```python
from build123d import *

# Parameters (mm, degrees)
SKETCH_W    = 80
SKETCH_H    = 88
SKETCH_R    = 9.5
SKETCH_R_2  = 3
PAD_DEPTH   = 10
FILLET_R    = 1
FILLET001_R = 10


with BuildPart() as part:
    # Sketch → Pad (new body)
    with BuildSketch(Plane.XY):
        with Locations((15, -15)):
            Rectangle(SKETCH_W, SKETCH_H)
        with Locations((0, -30)):
            Circle(SKETCH_R, mode=Mode.SUBTRACT)
        with Locations((-10, -52)):
            Circle(SKETCH_R_2, mode=Mode.SUBTRACT)
        with Locations((40, -52)):
            Circle(SKETCH_R_2, mode=Mode.SUBTRACT)
        with Locations((40, 22)):
            Circle(SKETCH_R_2, mode=Mode.SUBTRACT)
        with Locations((-10, 22)):
            Circle(SKETCH_R_2, mode=Mode.SUBTRACT)
        with BuildLine():
            ThreePointArc((-5, -6.244998), (8, 0), (-5, 6.244998))
            Line((-5, 9), (-5, 6.244998))
            Line((-8.125, 9), (-5, 9))
            Line((-8.125, -9), (-8.125, 9))
            Line((-5, -9), (-8.125, -9))
            Line((-5, -6.244998), (-5, -9))
        make_face(mode=Mode.SUBTRACT)
    extrude(amount=PAD_DEPTH)

    # Fillet
    fillet_edges = [part.edges().sort_by_distance(p)[0] for p in [
        (55, -59, 5),
        (55, 29, 5),
    ]]
    fillet(fillet_edges, radius=FILLET_R)

    # Fillet001
    fillet001_edges = [part.edges().sort_by_distance(p)[0] for p in [
        (-25, -59, 5),
        (-25, 29, 5),
    ]]
    fillet(fillet001_edges, radius=FILLET001_R)


solid = part.part
```
The model under review builds one solid part; all positions refer to its coordinate system, in mm. A direction names the side the tool comes from. Coordinates: 2 decimals unless noted, no trailing zeros. Write each loop counter-clockwise with the first axis right and the second up, starting at its lowest first coordinate (ties: lowest second). Pieces come first, ordered by that corner, then holes. Notation, with made-up numbers: (53, 19) -> (62, 19) arc R19 ccw to (62, 44) -> close; hole circle Ø9 at (-20, 70.5). An arc over 180 degrees is marked (long way). One line per item, written item: value. Start each with the question number.
Q1. Add section A-A, the plane y = 0. Give the boundary of the cut face in (x, z) (3 decimals), then the cut area to 3 significant figures.
Q2. To check wall thickness, follow probe 1 along Y at (x, z) = (0, 7); probe 2 along Y at (x, z) = (-4, 4.5); probe 3 along X at (y, z) = (0, 3.25) (3 decimals). State the ranges of each line that lie inside material, in increasing order.
Q3. Add section B-B, the plane x = 40. Give the boundary of the cut face in (y, z), then the cut area to 3 significant figures.
Q4. Add section D-D, the plane y = 22. Give the boundary of the cut face in (x, z), then the cut area to 3 significant figures.
Q5. Add section C-C, the plane z = 5.75. Give the boundary of the cut face in (x, y) (3 decimals).
Q6. Clearance check with a flat-ended pin moving along its axis: P1, Ø9.5, axis at x = 40, y = 22, coming from the -Z side. State where the tip first meets the part, or that it passes through.
Q7. The part is to be moulded in two halves that separate along X. For faces 1 (the face through (55, -16, 5)), 2 (the face through (-22.15, 25.99, 5.07)), 3 (the face through (14, -14, 0)), 4 (the face through (37.79, -49.97, 4.93)), say which applies: +X half, -X half, draft (parallel to the pull), parting line (faces both ways), or undercut.
Q8. For faces 5 (the face through (-5, -8, 5)), 6 (the face through (19, 29, 5)), list the 3-axis set-ups (+Z, -Z, +X, -X, +Y, -Y) from which the entire face can be reached by the end or side of a thin tool; tool diameter is ignored.
Response:
1. outline: (-25, 0) -> (-8.125, 0) -> (-8.125, 10) -> (-25, 10) -> close; (8, 0) -> (55, 0) -> (55, 10) -> (8, 10) -> close
1. area: 639 mm²
2. probe 1: -59 to -39.5, -20.5 to -8, 8 to 29
2. probe 2: -59 to -38.62, -21.38 to -6.93, 6.93 to 29
2. probe 3: -25 to -8.125, 8 to 55
3. outline: (-59, 0) -> (-55, 0) -> (-55, 10) -> (-59, 10) -> close; (-49, 0) -> (19, 0) -> (19, 10) -> (-49, 10) -> close; (25, 0) -> (29, 0) -> (29, 10) -> (25, 10) -> close
3. area: 760 mm²
4. outline: (-24.54, 0) -> (-13, 0) -> (-13, 10) -> (-24.54, 10) -> close; (-7, 0) -> (37, 0) -> (37, 10) -> (-7, 10) -> close; (43, 0) -> (55, 0) -> (55, 10) -> (43, 10) -> close
4. area: 675 mm²
5. outline: (-25, -49) arc R10 ccw to (-15, -59) -> (54, -59) arc R1 ccw to (55, -58) -> (55, 28) arc R1 ccw to (54, 29) -> (-15, 29) arc R10 ccw to (-25, 19) -> close; hole circle Ø6 at (-10, -52); hole circle Ø6 at (-10, 22); hole circle Ø19 at (0, -30); hole (-8.125, -9) -> (-5, -9) -> (-5, -6.245) arc R8 ccw (long way) to (-5, 6.245) -> (-5, 9) -> (-8.125, 9) -> close; hole circle Ø6 at (40, -52); hole circle Ø6 at (40, 22)
6. P1: z = 0
7. face 1: +X half
7. face 2: -X half
7. face 3: draft
7. face 4: undercut
8. face 5: +Z, -Z
8. face 6: +Z, -Z, +X, -X, +Y
